```python
from build123d import *

# Parameters (mm, degrees)
F1_DEPTH = 10
F2_DEPTH = 3.5
F3_SIZE  = 0.1


with BuildPart() as f1:
    # F0 (on Top) → F1 (new body)
    with BuildSketch(Plane.XY):
        Polygon((39.232051, 0), (19.616025, 33.975953), (-19.616025, 33.975953), (-39.232051, 0), (-19.616025, -33.975953), (19.616025, -33.975953), align=None)
        Polygon((-18.75, 32.475953), (18.75, 32.475953), (37.5, 0), (18.75, -32.475953), (-18.75, -32.475953), (-37.5, 0), align=None, mode=Mode.SUBTRACT)
    extrude(amount=F1_DEPTH)

    # F0 (on Top) → F2 (join)
    with BuildSketch(Plane.XY):
        Polygon((43.273503, 0), (21.636751, 37.475953), (-21.636751, 37.475953), (-43.273503, 0), (-21.636751, -37.475953), (21.636751, -37.475953), align=None)
        Polygon((-19.616025, 33.975953), (19.616025, 33.975953), (39.232051, 0), (19.616025, -33.975953), (-19.616025, -33.975953), (-39.232051, 0), align=None, mode=Mode.SUBTRACT)
    extrude(amount=F2_DEPTH)

    # F3
    f3_edges = [f1.edges().sort_by_distance(p)[0] for p in [
        (0, -37.475953, 0),
        (32.455127, -18.737976, 0),
        (32.455127, 18.737976, 0),
        (0, 37.475953, 0),
        (-32.455127, 18.737976, 0),
        (-32.455127, -18.737976, 0),
        (-28.125, -16.237976, 0),
        (-28.125, 16.237976, 0),
        (0, 32.475953, 0),
        (28.125, 16.237976, 0),
        (28.125, -16.237976, 0),
        (0, -32.475953, 0),
        (29.424038, 16.987976, 10),
        (0, 33.975953, 10),
        (-29.424038, 16.987976, 10),
        (-29.424038, -16.987976, 10),
        (0, -33.975953, 10),
        (29.424038, -16.987976, 10),
        (0, 32.475953, 10),
        (28.125, 16.237976, 10),
        (28.125, -16.237976, 10),
        (0, -32.475953, 10),
        (-28.125, -16.237976, 10),
        (-28.125, 16.237976, 10),
    ]]
    chamfer(f3_edges, length=F3_SIZE)


solid = f1.part
```
Verification items for the finished model (mm, model axes). A direction names the side the tool comes from. Give positions to 0.01 mm unless a question says otherwise; leave off trailing zeros. Order: outer loops, then holes, each group sorted by start corner. A loop starts at its lowest first (then second) coordinate and runs counter-clockwise, first axis right, second up. Notation, with made-up numbers: M -29.5,61 L 24.5,61 A15 ccw 24.5,89 Z; hole C 61,-20 d5. An arc over 180 degrees is marked long. Return JSON: item names as keys, results as strings. Group by question number.
1) Section check B-B on z = 7.25. Record the cut outline in (x, y).
2) Access from +Z, -Z, +X, -X, +Y, -Y to the whole of each face (thin tool, end or side, straight path). Record for faces 1 (the face through (0, 33.976, 7)), 2 (the face through (-29.56, -16.75, 6.66)), 3 (the face through (0, -37.476, 2)).
3) Mould release check, pull along X, two halves, no side actions. Record for faces 4 (the face through (0, -32.476, 5)), 5 (the face through (-29.3, 17.2, 6.7)), 6 (the face through (32.304, -19, 1.776)): pulls with the +X half, pulls with the -X half, needs draft (parallel to the pull), parting line crosses it, or undercut.
4) Section check A-A on x = 4. Record the cut outline in (y, z), and give its area (3 significant figures).
5) Go/stop test with flat-tipped pins: pin 1 Ø2 at (x, z) = (29, 5) entering from -Y; pin 2 Ø2 at (y, z) = (13.5, 3.5) entering from -X; pin 3 Ø3 at (x, z) = (-3, 8) entering from -Y; pin 4 Ø5 at (x, y) = (-21.5, -19) entering from +Z. Record where each tip stops, or that it passes through.
6) Section check D-D on z = 2.5. Record the cut outline in (x, y), and give its area (3 significant figures).
7) Scan lines: line 1 (Y direction, x = -16.5, z = 2.25); line 2 (Y direction, x = 9, z = 5.25); line 3 (X direction, y = 12.5, z = 1). Record each from-to range of solid material in increasing order.
8) Section check C-C on y = -29. Record the cut outline in (x, z).
Answer block:
{
 "1": {"outline": "M -39.23,0 L -19.62,-33.98 L 19.62,-33.98 L 39.23,0 L 19.62,33.98 L -19.62,33.98 Z; hole M -37.5,0 L -18.75,-32.48 L 18.75,-32.48 L 37.5,0 L 18.75,32.48 L -18.75,32.48 Z"},
 "2": {"face 1": "+Z, +X, -X, +Y", "face 2": "+Z, -X, -Y", "face 3": "+Z, -Z, +X, -X, -Y"},
 "3": {"face 4": "undercut", "face 5": "pulls with the -X half", "face 6": "pulls with the +X half"},
 "4": {"outline": "M -37.48,0.1 L -37.38,0 L -32.58,0 L -32.48,0.1 L -32.48,9.9 L -32.58,10 L -33.88,10 L -33.98,9.9 L -33.98,3.5 L -37.48,3.5 Z; M 32.48,0.1 L 32.58,0 L 37.38,0 L 37.48,0.1 L 37.48,3.5 L 33.98,3.5 L 33.98,9.9 L 33.88,10 L 32.58,10 L 32.48,9.9 Z", "area": "54.5 mm^2"},
 "5": {"pin 1": "stops at y = -19.45", "pin 2": "stops at x = -36.06", "pin 3": "stops at y = -33.98", "pin 4": "passes through"},
 "6": {"outline": "M -43.27,0 L -21.64,-37.48 L 21.64,-37.48 L 43.27,0 L 21.64,37.48 L -21.64,37.48 Z; hole M -37.5,0 L -18.75,-32.48 L 18.75,-32.48 L 37.5,0 L 18.75,32.48 L -18.75,32.48 Z", "area": "1,210 mm^2"},
 "7": {"line 1": "y = -37.48 to -32.48, 32.48 to 37.48", "line 2": "y = -33.98 to -32.48, 32.48 to 33.98", "line 3": "x = -36.06 to -30.28, 30.28 to 36.06"},
 "8": {"outline": "M -26.53,0.1 L -26.41,0 L -20.87,0 L -20.76,0.1 L -20.76,9.9 L -20.87,10 L -22.37,10 L -22.49,9.9 L -22.49,3.5 L -26.53,3.5 Z; M 20.76,0.1 L 20.87,0 L 26.41,0 L 26.53,0.1 L 26.53,3.5 L 22.49,3.5 L 22.49,9.9 L 22.37,10 L 20.87,10 L 20.76,9.9 Z"}
}
